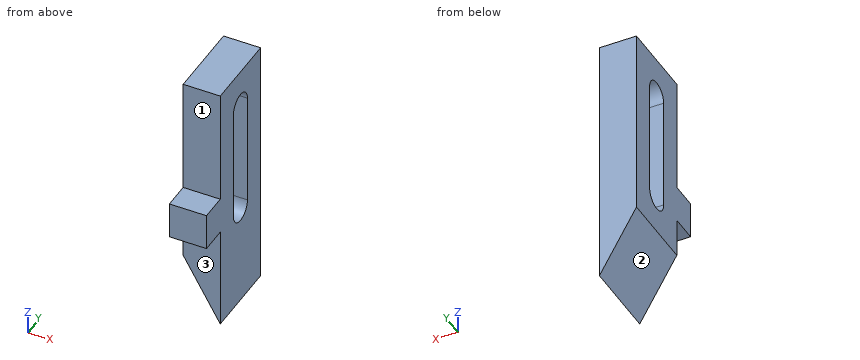
```python
from build123d import *

# Parameters (mm, degrees)
BOSS_EXTRUDE1_DEPTH = 19
CUT_EXTRUDE1_DEPTH  = 10
SKETCH4_W           = 9
SKETCH4_H           = 9
BOSS_EXTRUDE2_DEPTH = 6.5


with BuildPart() as part:
    # Sketch1 → Boss-Extrude1 (new body)
    with BuildSketch(Plane(origin=(0, 0, 0), x_dir=(1, 0, 0), z_dir=(0, 1, 0))):
        Polygon((15.5, 26.846787517), (15.5, -20), (24.5, -20), (24.5, 42.435244785), align=None)
    extrude(amount=BOSS_EXTRUDE1_DEPTH)

    # Sketch3 → Cut-Extrude1 (cut, through all)
    with BuildSketch(Plane.ZY.offset(-15.5)):
        with BuildLine():
            Line((-17.346787517, 12.8), (10.5, 12.8))
            ThreePointArc((10.5, 12.8), (13.8, 9.5), (10.5, 6.2))
            Line((10.5, 6.2), (-17.346787517, 6.2))
            ThreePointArc((-17.346787517, 6.2), (-20.646787517, 9.5), (-17.346787517, 12.8))
        make_face()
    extrude(amount=-CUT_EXTRUDE1_DEPTH, mode=Mode.SUBTRACT)

    # Sketch4 → Boss-Extrude2 (add)
    with BuildSketch(Plane.XZ):
        with Locations((20, -12.75)):
            Rectangle(SKETCH4_W, SKETCH4_H)
    extrude(amount=BOSS_EXTRUDE2_DEPTH)


solid = part.part
```
Read the model definition and answer for the solid it produces. Units are mm, in the model's axes. Face numbers are marked on the shaded views. A direction names the side the tool comes from. Coordinates: 2 decimals unless noted, no trailing zeros. Write each loop counter-clockwise with the first axis right and the second up, starting at its lowest first coordinate (ties: lowest second). Pieces come first, ordered by that corner, then holes. Notation, with made-up numbers: (29.5, 0.25) - (44.5, 0.25) arc R29 ccw to (44.5, 20.25) - close; hole circle Ø1 at (33.5, 56). An arc over 180 degrees is marked (long way). Answer as a JSON object with one key per item and string values. Group by question number.
1. A cutting plane is placed at A-A (y = 9.5). Determine the outline of the cut face in (x, z).
2. A cutting plane is placed at D-D (z = -23.5). Determine the outline of the cut face in (x, y).
3. A cutting plane is placed at C-C (x = 21.5). Determine the outline of the cut face in (y, z), plus the area to 3 significant figures.
4. Consider L1, parallel to Y at x = 24, z = -5; L2, parallel to Y at x = 17.75, z = -8.5; L3, parallel to Z at x = 22, y = -3. Determine where each line is inside the solid, lowest interval first. Write a range as [from, to].
5. Each of these flat-tipped pins is pushed along its axis until it touches: P1, Ø2, axis at x = 21.5, y = -2, coming from the -Z side; P2, Ø2.5, axis at x = 21, z = -34, coming from the -Y side. Where does it stop, or does it pass through?
6. A cutting plane is placed at B-B (z = 5.5). Determine the outline of the cut face in (x, y), plus the area to 3 significant figures.
7. Which of the six approach directions +Z, -Z, +X, -X, +Y, -Y give full straight-line access (tool end or side, diameter ignored) to the marked faces 1, 2 and 3?
Worked out:
{
 "1": {"outline": "(15.5, -26.85) - (24.5, -42.44) - (24.5, -20.65) - (15.5, -20.65) - close; (15.5, 13.8) - (24.5, 13.8) - (24.5, 20) - (15.5, 20) - close"},
 "2": {"outline": "(15.5, 0) - (24.5, 0) - (24.5, 19) - (15.5, 19) - close"},
 "3": {"outline": "(-6.5, -17.25) - (0, -17.25) - (0, -37.24) - (19, -37.24) - (19, 20) - (0, 20) - (0, -8.25) - (-6.5, -8.25) - close; hole (6.2, -17.35) arc R3.3 ccw to (12.8, -17.35) - (12.8, 10.5) arc R3.3 ccw to (6.2, 10.5) - close", "area": "928 mm²"},
 "4": {"L1": "y = [0, 6.2], [12.8, 19]", "L2": "y = [-6.5, 6.2], [12.8, 19]", "L3": "z = [-17.25, -8.25]"},
 "5": {"P1": "stops at z = -17.25", "P2": "stops at y = 0"},
 "6": {"outline": "(15.5, 0) - (24.5, 0) - (24.5, 6.2) - (15.5, 6.2) - close; (15.5, 12.8) - (24.5, 12.8) - (24.5, 19) - (15.5, 19) - close", "area": "112 mm²"},
 "7": {"face 1": "+Z, +X, -X, -Y", "face 2": "-Z, -X, +Y, -Y", "face 3": "-Z, +X, -X, -Y"}
}
